from build123d import *

# Parameters (mm, degrees)
F0_W     = 50
F0_H     = 50
F0_R     = 3
F0_W_2   = 4.7625
F0_H_2   = 4.7625
F1_DEPTH = 10


with BuildPart() as f1:
    # F0 (on Top) → F1 (new body)
    with BuildSketch(Plane.XY):
        with Locations((25, -25)):
            Rectangle(F0_W, F0_H)
        with Locations((5, -45)):
            Circle(F0_R, mode=Mode.SUBTRACT)
        with Locations((25, -25)):
            Rectangle(F0_W_2, F0_H_2, mode=Mode.SUBTRACT)
        with Locations((45, -5)):
            Circle(F0_R, mode=Mode.SUBTRACT)
    extrude(amount=F1_DEPTH)


solid = f1.part
Can you work these out from the model? Positions are in its coordinate system, mm. A direction names the side the tool comes from. Round coordinates to 2 decimals unless told otherwise and drop trailing zeros. Write each loop counter-clockwise with the first axis right and the second up, starting at its lowest first coordinate (ties: lowest second). Pieces come first, ordered by that corner, then holes. Notation, with made-up numbers: (60, -14) -> (89, -14) arc R22 ccw to (89, 8) -> close; hole circle Ø6 at (71.5, -7). An arc over 180 degrees is marked (long way). One line per question, with ' | ' between items. Start each with the question number.
1) Suppose I cut it at C-C on y = -5. Write out the boundary of the cut face in (x, z), then the cut area to 3 significant figures.
2) If we mould it in two halves opening along X, with no side actions, what happens to faces 1 (the flat face through (50, -25, 5)), 2 (the cylindrical face through (42, -5, 5)), 3 (the flat face through (19, -25, 10))? For each: released by +X, released by -X, zero draft, split by the parting line, or undercut.
3) Suppose I cut it at B-B on z = 5. Write out the boundary of the cut face in (x, y).
4) I need wall thicknesses on line 1 (Y direction, x = 26.5, z = 7.75); line 2 (Y direction, x = 45, z = 3.25); line 3 (X direction, y = -24.5, z = 3.5). Which ranges of each line are inside material? Lowest first, please. Write a range as [from, to].
5) Suppose I cut it at A-A on x = 45. Write out the boundary of the cut face in (y, z).
6) On a 3-axis mill with a long thin cutter (end or side, diameter ignored), from which of +Z, -Z, +X, -X, +Y, -Y can I reach the whole of each face in a straight line? I mean faces 4 (the flat face through (0, -25, 5)), 5 (the flat face through (25, -22.619, 5)). Say none if no direction works.
7) I'm going to push a flat-ended pin straight in: P1, Ø5, axis at x = 5, y = -45, coming from the -Z side. Where does the tip first touch, or does it pass through?
Return value:
1) outline: (0, 0) -> (42, 0) -> (42, 10) -> (0, 10) -> close; (48, 0) -> (50, 0) -> (50, 10) -> (48, 10) -> close | area: 440 mm2
2) face 1: released by +X | face 2: undercut | face 3: zero draft
3) outline: (0, -50) -> (50, -50) -> (50, 0) -> (0, 0) -> close; hole circle Ø6 at (5, -45); hole (22.62, -27.38) -> (27.38, -27.38) -> (27.38, -22.62) -> (22.62, -22.62) -> close; hole circle Ø6 at (45, -5)
4) line 1: y = [-50, -27.38], [-22.62, 0] | line 2: y = [-50, -8], [-2, 0] | line 3: x = [0, 22.62], [27.38, 50]
5) outline: (-50, 0) -> (-8, 0) -> (-8, 10) -> (-50, 10) -> close; (-2, 0) -> (0, 0) -> (0, 10) -> (-2, 10) -> close
6) face 4: +Z, -Z, -X, +Y, -Y | face 5: +Z, -Z
7) P1: passes through
